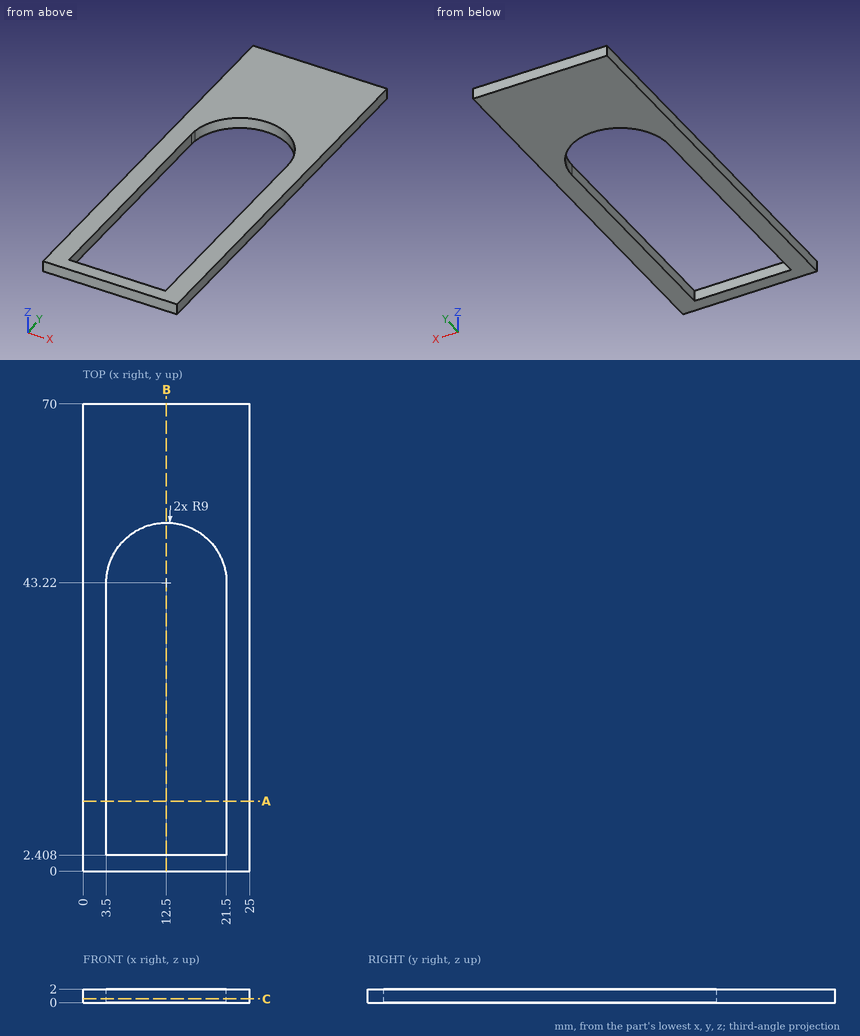
The figure shows three views and two pictorial views of one solid part (mm, origin at its lowest corner). Answer the questions. Round coordinates to 2 decimals unless told otherwise and drop trailing zeros. Loops run counter-clockwise (first coordinate to the right, second up) from the corner with the lowest first, then second, coordinate; pieces in that order, holes last. Notation, with made-up numbers: (-8, 82.5) - (10, 82.5) arc R23 ccw to (10, 93.5) - close; hole circle Ø9 at (-3.5, 18.5). An arc over 180 degrees is marked (long way). Use one line per item in the form item = value. Start each with the question number.
(1) Find section C-C on z = 0.55. Determine the outline of the cut face in (x, y).
(2) Consider line 1 (X direction, y = 34, z = 0.6); line 2 (Y direction, x = 13, z = 1.5); line 3 (X direction, y = 51.5, z = 1.05) (1 decimal). Determine where each line is inside the solid, lowest interval first.
(3) Find section B-B on x = 12.5. Determine the outline of the cut face in (y, z).
(4) Find section A-A on y = 10.5. Determine the outline of the cut face in (x, z), and give its area (3 significant figures).
Answer list:
q1.outline = (0, 0) - (25, 0) - (25, 70) - (0, 70) - close; hole (3.5, 2.41) - (21.5, 2.41) - (21.5, 43.22) arc R9 ccw to (3.56, 44.23) arc R9 ccw to (3.5, 43.22) - close
q2.line_1 = 0 to 3.5, 21.5 to 25
q2.line_2 = 0 to 2.41, 52.21 to 70
q2.line_3 = 0 to 9, 16 to 25
q3.outline = (0, 0) - (2.41, 0) - (2.41, 2) - (0, 2) - close; (52.22, 0) - (70, 0) - (70, 2) - (52.22, 2) - close
q4.outline = (0, 0) - (3.5, 0) - (3.5, 2) - (0, 2) - close; (21.5, 0) - (25, 0) - (25, 2) - (21.5, 2) - close
q4.area = 14.0 mm^2
